from build123d import *

# Parameters (mm, degrees)
SKETCH_1_W             = 120
SKETCH_1_H             = 50
EXTRUDE_1_DEPTH        = 15
SKETCH_2_R             = 6
CUT_EXTRUDE_1_DEPTH    = 8
SKETCH_3_R             = 11
CUT_EXTRUDE_2_DEPTH    = 8
SKETCH_10_R            = 3.25
CUT_EXTRUDE_4_DEPTH    = 10
SKETCH_11_R            = 5
CUT_EXTRUDE_5_DEPTH    = 10
HOLE_WIZARD_M3_1_D     = 2.5
HOLE_WIZARD_M3_1_DEPTH = 5
HOLE_WIZARD_M3_1_TIP   = 0.751075774
HOLE_WIZARD_M3_2_D     = 2.5
HOLE_WIZARD_M3_2_DEPTH = 5
HOLE_WIZARD_M3_2_TIP   = 0.751075774


with BuildPart() as part:
    # 草图1 → 凸台-拉伸1 (new body)
    with BuildSketch(Plane.XY):
        Rectangle(SKETCH_1_W, SKETCH_1_H)
    extrude(amount=EXTRUDE_1_DEPTH)

    # 草图2 → 切除-拉伸1 (cut)
    with BuildSketch(Plane.XY.offset(15)):
        with Locations((-35, 0)):
            Circle(SKETCH_2_R)
        with Locations((35, 0)):
            Circle(SKETCH_2_R)
    extrude(amount=-CUT_EXTRUDE_1_DEPTH, mode=Mode.SUBTRACT)

    # 草图3 → 切除-拉伸2 (cut)
    with BuildSketch(Plane.XY.offset(15)):
        Circle(SKETCH_3_R)
    extrude(amount=-CUT_EXTRUDE_2_DEPTH, mode=Mode.SUBTRACT)

    # 草图10 → 切除-拉伸4 (cut)
    with BuildSketch(Plane.XY.offset(7)):
        with Locations((-35, 0)):
            Circle(SKETCH_10_R)
        with Locations((35, 0)):
            Circle(SKETCH_10_R)
    extrude(amount=-CUT_EXTRUDE_4_DEPTH, mode=Mode.SUBTRACT)

    # 草图11 → 切除-拉伸5 (cut)
    with BuildSketch(Plane.XY.offset(7)):
        Circle(SKETCH_11_R)
    extrude(amount=-CUT_EXTRUDE_5_DEPTH, mode=Mode.SUBTRACT)

    # M3 螺纹孔1
    with Locations(Plane(origin=(0, 25, 0), x_dir=(1, 0, 0), z_dir=(0, 1, 0))):
        with Locations((30, -7.5), (-30, -7.5)):
            Hole(HOLE_WIZARD_M3_1_D / 2, depth=HOLE_WIZARD_M3_1_DEPTH)
            with Locations((0, 0, -(HOLE_WIZARD_M3_1_DEPTH + HOLE_WIZARD_M3_1_TIP / 2))):  # 118° drill point
                Cone(0, HOLE_WIZARD_M3_1_D / 2, HOLE_WIZARD_M3_1_TIP, mode=Mode.SUBTRACT)

    # M3 螺纹孔2
    with Locations(Plane(origin=(0, -25, 0), x_dir=(-1, 0, 0), z_dir=(0, -1, 0))):
        with Locations((-30, -7.5), (30, -7.5)):
            Hole(HOLE_WIZARD_M3_2_D / 2, depth=HOLE_WIZARD_M3_2_DEPTH)
            with Locations((0, 0, -(HOLE_WIZARD_M3_2_DEPTH + HOLE_WIZARD_M3_2_TIP / 2))):  # 118° drill point
                Cone(0, HOLE_WIZARD_M3_2_D / 2, HOLE_WIZARD_M3_2_TIP, mode=Mode.SUBTRACT)


solid = part.part
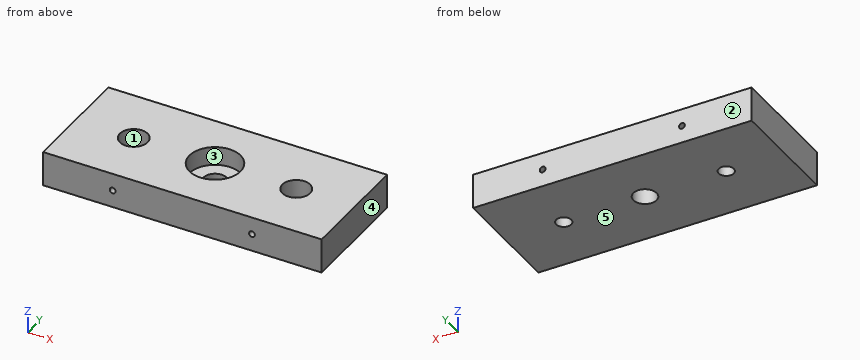
Check sheet for the modelled part. Datum: model origin and axes. Units: mm. Face numbers are marked on the shaded views. A direction names the side the tool comes from. Give positions to 0.01 mm unless a question says otherwise; leave off trailing zeros. Loops run counter-clockwise (first coordinate to the right, second up) from the corner with the lowest first, then second, coordinate; pieces in that order, holes last. Notation, with made-up numbers: M 37.5,2 L 55.5,2 A9 ccw 55.5,6 Z; hole C 34.25,-27.75 d9. An arc over 180 degrees is marked long. Use a Markdown table: item, result. Add a question column.
Q1. Sectioned sample at C-C, the plane z = 12. Record the cut outline in (x, y), then the cut area to 3 significant figures.
Q2. Sectioned sample at A-A, the plane x = 35. Record the cut outline in (y, z), then the cut area to 4 significant figures.
Q3. Go/stop test with flat-tipped pins: pin 1 (17.5 mm diameter, centred on x = 0, y = 0, fed in from +Z); pin 2 (1.5 mm diameter, centred on x = -30, z = 7.5, fed in from +Y); pin 3 (2 mm diameter, centred on x = -30, z = 7.5, fed in from +Y); pin 4 (4 mm diameter, centred on x = -35, y = 0, fed in from -Z). Record where each tip stops, or that it passes through.
Q4. Tool access check on the marked faces 1 and 2. Record the directions out of +Z, -Z, +X, -X, +Y, -Y that give a thin tool (end or side, any length) a straight path to the whole face; none if there is none.
Q5. Mould release check, pull along X, two halves, no side actions. Record for the marked faces 3, 4 and 5: pulls with the +X half, pulls with the -X half, needs draft (parallel to the pull), parting line crosses it, or undercut.
Q6. Sectioned sample at D-D, the plane x = 0. Record the cut outline in (y, z).
Q7. Sectioned sample at B-B, the plane y = 0. Record the cut outline in (x, z), then the cut area to 3 significant figures.
Q8. Scan lines: line 1 along X through (y, z) = (23.65, 7.5); line 2 along Y through (x, z) = (0, 11); line 3 along Y through (x, z) = (0, 2.5). Record each from-to range of solid material in increasing order. Write a range as [from, to].
Verdict:
| question | item | result |
|---|---|---|
| 1 | outline | M -60,-25 L 60,-25 L 60,25 L -60,25 Z; hole C -35,0 d12; hole C 0,0 d22; hole C 35,0 d12 |
| 1 | area | 5,390 mm^2 |
| 2 | outline | M -25,0 L -3.25,0 L -3.25,7 L -6,7 L -6,15 L -25,15 Z; M 3.25,0 L 25,0 L 25,15 L 6,15 L 6,7 L 3.25,7 Z |
| 2 | area | 608.5 mm^2 |
| 3 | pin 1 | z = 7 |
| 3 | pin 2 | y = 19.7 |
| 3 | pin 3 | y = 19.85 |
| 3 | pin 4 | through |
| 4 | face 1 | +Z |
| 4 | face 2 | +Z, -Z, +X, -X, +Y |
| 5 | face 3 | undercut |
| 5 | face 4 | pulls with the +X half |
| 5 | face 5 | needs draft |
| 6 | outline | M -25,0 L -5,0 L -5,7 L -11,7 L -11,15 L -25,15 Z; M 5,0 L 25,0 L 25,15 L 11,15 L 11,7 L 5,7 Z |
| 7 | outline | M -60,0 L -38.25,0 L -38.25,7 L -41,7 L -41,15 L -60,15 Z; M -31.75,0 L -5,0 L -5,7 L -11,7 L -11,15 L -29,15 L -29,7 L -31.75,7 Z; M 5,0 L 31.75,0 L 31.75,7 L 29,7 L 29,15 L 11,15 L 11,7 L 5,7 Z; M 38.25,0 L 60,0 L 60,15 L 41,15 L 41,7 L 38.25,7 Z |
| 7 | area | 1,270 mm^2 |
| 8 | line 1 | [-60, -31.25], [-28.75, 28.75], [31.25, 60] |
| 8 | line 2 | [-25, -11], [11, 25] |
| 8 | line 3 | [-25, -5], [5, 25] |
